```python
from build123d import *

# Parameters (mm, degrees)
SKETCH1_W                    = 152.4
SKETCH1_H                    = 152.4
EXTRUDE1_DEPTH               = 9.525
CUT_EXTRUDE1_DEPTH           = 10.525
F_10_32_TAPPED_HOLE1_D       = 4.0386
F_10_32_TAPPED_HOLE1_DEPTH   = 13.6144
F_10_32_TAPPED_HOLE1_TIP     = 1.213317848
SKETCH5_R                    = 4.09575
CUT_EXTRUDE2_DEPTH           = 10.525
F_5_16_18_TAPPED_HOLE1_D     = 6.5278
F_5_16_18_TAPPED_HOLE1_DEPTH = 22.9362
F_5_16_18_TAPPED_HOLE1_TIP   = 1.961148974


with BuildPart() as part:
    # Sketch1 → Extrude1 (new body)
    with BuildSketch(Plane(origin=(0, 0, 0), x_dir=(1, 0, 0), z_dir=(0, 1, 0))):
        with Locations((76.2, 76.2)):
            Rectangle(SKETCH1_W, SKETCH1_H)
    extrude(amount=EXTRUDE1_DEPTH)

    # Sketch2 → Cut-Extrude1 (cut, through all)
    with BuildSketch(Plane(origin=(0, 9.525, 0), x_dir=(1, 0, 0), z_dir=(0, 1, 0))):
        with BuildLine():
            Line((141.2875, 33.3248), (138.1125, 33.3248))
            ThreePointArc((138.1125, 33.3248), (134.744903955, 34.719703955), (133.35, 38.0873))
            Line((133.35, 38.0873), (133.35, 38.1127))
            ThreePointArc((133.35, 38.1127), (134.744903955, 41.480296045), (138.1125, 42.8752))
            Line((138.1125, 42.8752), (141.2875, 42.8752))
            ThreePointArc((141.2875, 42.8752), (144.655096045, 41.480296045), (146.05, 38.1127))
            Line((146.05, 38.1127), (146.05, 38.0873))
            ThreePointArc((146.05, 38.0873), (144.655096045, 34.719703955), (141.2875, 33.3248))
        make_face()
        with BuildLine():
            Line((19.05, 38.0873), (19.05, 38.1127))
            ThreePointArc((19.05, 38.1127), (17.655096045, 41.480296045), (14.2875, 42.8752))
            Line((14.2875, 42.8752), (11.1125, 42.8752))
            ThreePointArc((11.1125, 42.8752), (7.744903955, 41.480296045), (6.35, 38.1127))
            Line((6.35, 38.1127), (6.35, 38.0873))
            ThreePointArc((6.35, 38.0873), (7.744903955, 34.719703955), (11.1125, 33.3248))
            Line((11.1125, 33.3248), (14.2875, 33.3248))
            ThreePointArc((14.2875, 33.3248), (17.655096045, 34.719703955), (19.05, 38.0873))
        make_face()
        with BuildLine():
            Line((11.1125, 80.9752), (14.2875, 80.9752))
            ThreePointArc((14.2875, 80.9752), (17.655096045, 79.580296045), (19.05, 76.2127))
            Line((19.05, 76.2127), (19.05, 76.1873))
            ThreePointArc((19.05, 76.1873), (17.655096045, 72.819703955), (14.2875, 71.4248))
            Line((14.2875, 71.4248), (11.1125, 71.4248))
            ThreePointArc((11.1125, 71.4248), (7.744903955, 72.819703955), (6.35, 76.1873))
            Line((6.35, 76.1873), (6.35, 76.2127))
            ThreePointArc((6.35, 76.2127), (7.744903955, 79.580296045), (11.1125, 80.9752))
        make_face()
        with BuildLine():
            Line((133.35, 76.2127), (133.35, 76.1873))
            ThreePointArc((133.35, 76.1873), (134.744903955, 72.819703955), (138.1125, 71.4248))
            Line((138.1125, 71.4248), (141.2875, 71.4248))
            ThreePointArc((141.2875, 71.4248), (144.655096045, 72.819703955), (146.05, 76.1873))
            Line((146.05, 76.1873), (146.05, 76.2127))
            ThreePointArc((146.05, 76.2127), (144.655096045, 79.580296045), (141.2875, 80.9752))
            Line((141.2875, 80.9752), (138.1125, 80.9752))
            ThreePointArc((138.1125, 80.9752), (134.744903955, 79.580296045), (133.35, 76.2127))
        make_face()
    extrude(amount=-CUT_EXTRUDE1_DEPTH, mode=Mode.SUBTRACT)

    # #10-32 Tapped Hole1
    with Locations(Plane(origin=(0, 9.525, 0), x_dir=(-1, 0, 0), z_dir=(0, 1, 0))):
        with Locations((-44.45, -107.95), (-107.95, -107.95), (-107.95, -133.35), (-44.45, -133.35)):
            Hole(F_10_32_TAPPED_HOLE1_D / 2, depth=F_10_32_TAPPED_HOLE1_DEPTH)
            with Locations((0, 0, -(F_10_32_TAPPED_HOLE1_DEPTH + F_10_32_TAPPED_HOLE1_TIP / 2))):  # 118° drill point
                Cone(0, F_10_32_TAPPED_HOLE1_D / 2, F_10_32_TAPPED_HOLE1_TIP, mode=Mode.SUBTRACT)

    # Sketch5 → Cut-Extrude2 (cut, through all)
    with BuildSketch(Plane(origin=(0, 9.525, 0), x_dir=(1, 0, 0), z_dir=(0, 1, 0))):
        with Locations(Location((57.15, 95.25, 0), (0, 0, 270))):  # turned: the seam where the file's is
            Circle(SKETCH5_R)
        with Locations(Location((95.25, 95.25, 0), (0, 0, 90))):  # turned: the seam where the file's is
            Circle(SKETCH5_R)
        with Locations(Location((57.15, 57.15, 0), (0, 0, 90))):  # turned: the seam where the file's is
            Circle(SKETCH5_R)
        with Locations(Location((95.25, 57.15, 0), (0, 0, 270))):  # turned: the seam where the file's is
            Circle(SKETCH5_R)
    extrude(amount=-CUT_EXTRUDE2_DEPTH, mode=Mode.SUBTRACT)

    # 5/16-18 Tapped Hole1
    with Locations(Plane(origin=(0, 9.525, 0), x_dir=(-1, 0, 0), z_dir=(0, 1, 0))):
        with Locations((-57.15, -76.2), (-95.25, -76.2)):
            Hole(F_5_16_18_TAPPED_HOLE1_D / 2, depth=F_5_16_18_TAPPED_HOLE1_DEPTH)
            with Locations((0, 0, -(F_5_16_18_TAPPED_HOLE1_DEPTH + F_5_16_18_TAPPED_HOLE1_TIP / 2))):  # 118° drill point
                Cone(0, F_5_16_18_TAPPED_HOLE1_D / 2, F_5_16_18_TAPPED_HOLE1_TIP, mode=Mode.SUBTRACT)


solid = part.part
```
Design review of the part built by this model. Coordinates are the model's own, in mm. A direction names the side the tool comes from. Coordinates: 2 decimals unless noted, no trailing zeros. Loops run counter-clockwise (first coordinate to the right, second up) from the corner with the lowest first, then second, coordinate; pieces in that order, holes last.
Q1. The part is to be moulded in two halves that separate along X. For faces 3 (the face through (75, 0, -77)), 4 (the face through (7.708, 4.829, -79.543)), say which applies: +X half, -X half, draft (parallel to the pull), parting line (faces both ways), or undercut.
Reported:
face 3: draft
face 4: undercut
Q2. Tool access review of faces 1 (the face through (144.618, 4.829, -72.783)), 2 (the face through (75, 5, 0)): name each direction out of +Z, -Z, +X, -X, +Y, -Y from which nothing blocks a thin tool from reaching the whole face with its end or side.
Reported:
face 1: +Y, -Y
face 2: +Z, +X, -X, +Y, -Y
Q3. We need section C-C on z = -95.25. State the section outline as (x, y) points (3 decimals).
Reported:
outline: (0, 0) - (53.054, 0) - (53.054, 9.525) - (0, 9.525) - close; (61.246, 0) - (91.154, 0) - (91.154, 9.525) - (61.246, 9.525) - close; (99.346, 0) - (152.4, 0) - (152.4, 9.525) - (99.346, 9.525) - close
Q4. To check wall thickness, follow line 1 (X direction, y = 5.75, z = -95.25); line 2 (X direction, y = 3.5, z = -133.35); line 3 (Z direction, x = 44.45, y = 7.25). State the ranges of each line that lie inside material, in increasing order.
Reported:
line 1: x = 0 to 53.05, 61.25 to 91.15, 99.35 to 152.4
line 2: x = 0 to 42.43, 46.47 to 105.93, 109.97 to 152.4
line 3: z = -152.4 to -135.37, -131.33 to -109.97, -105.93 to 0
Q5. We need section A-A on z = -133.35. State the section outline as (x, y) points (3 decimals).
Reported:
outline: (0, 0) - (42.431, 0) - (42.431, 9.525) - (0, 9.525) - close; (46.469, 0) - (105.931, 0) - (105.931, 9.525) - (46.469, 9.525) - close; (109.969, 0) - (152.4, 0) - (152.4, 9.525) - (109.969, 9.525) - close
Q6. We need section D-D on y = 2.75. State how many separate pieces and enclosed holes the cut face has, and give its area (3 significant figures).
Reported:
separate pieces: 1
enclosed holes: 14
area: 22,500 mm2
Q7. For pin 1 (10 mm diameter, centred on x = 21.5, z = -105, fed in from -Y), flat-tipped, find the tip position at first contact; note if it passes through.
Reported:
pin 1: stops at y = 0
Q8. We need section B-B on x = 57.15. State the section outline as (y, z) points (3 decimals).
Reported:
outline: (0, -152.4) - (9.525, -152.4) - (9.525, -99.346) - (0, -99.346) - close; (0, -91.154) - (9.525, -91.154) - (9.525, -79.464) - (0, -79.464) - close; (0, -72.936) - (9.525, -72.936) - (9.525, -61.246) - (0, -61.246) - close; (0, -53.054) - (9.525, -53.054) - (9.525, 0) - (0, 0) - close
